Work out the finished part from the listing and answer in its coordinate system (mm). A direction names the side the tool comes from. Coordinates: 2 decimals unless noted, no trailing zeros. Order: outer loops, then holes, each group sorted by start corner. A loop starts at its lowest first (then second) coordinate and runs counter-clockwise, first axis right, second up. Notation, with made-up numbers: M -28,-36 L 15,-36 A20 ccw 15,-15 Z; hole C 16,4.25 d5. An arc over 180 degrees is marked long. Use a Markdown table: item, result.
from build123d import *

# Parameters (mm, degrees)
F0_R     = 4
F0_R_2   = 2.25
F1_DEPTH = 4
F3_DEPTH = 2
F5_R     = 2
F6_R     = 3


with BuildPart() as f1:
    # F0 (on Top) → F1 (new body)
    with BuildSketch(Plane.XY):
        with Locations((-25, 75)):
            Circle(F0_R)
        with Locations((-25, 75)):
            Circle(F0_R_2, mode=Mode.SUBTRACT)
    extrude(amount=F1_DEPTH)


with BuildPart() as f1b:
    # F0 (on Top) → F1, piece 2 (new body)
    with BuildSketch(Plane.XY):
        with Locations((25, 75)):
            Circle(F0_R)
        with Locations((25, 75)):
            Circle(F0_R_2, mode=Mode.SUBTRACT)
    extrude(amount=F1_DEPTH)


with BuildPart() as f1c:
    # F0 (on Top) → F1, piece 3 (new body)
    with BuildSketch(Plane.XY):
        with Locations((-25, -75)):
            Circle(F0_R)
        with Locations((-25, -75)):
            Circle(F0_R_2, mode=Mode.SUBTRACT)
    extrude(amount=F1_DEPTH)


with BuildPart() as f1d:
    # F0 (on Top) → F1, piece 4 (new body)
    with BuildSketch(Plane.XY):
        with Locations((25, -75)):
            Circle(F0_R)
        with Locations((25, -75)):
            Circle(F0_R_2, mode=Mode.SUBTRACT)
    extrude(amount=F1_DEPTH)


with BuildPart() as f3:
    # F2 (on Top) → F3 (new body)
    with BuildSketch(Plane.XY):
        Polygon((-22.6102852702, 72.5742723009), (-25.4563351644, 71.6255890028), (-1.5811388301, 0), (0, 4.7434164903), align=None)
        Polygon((0, 4.7434164903), (-1.5811388301, 0), (0, -4.7434164903), (1.5811388301, 0), align=None)
        Polygon((0, -4.7434164903), (-1.5811388301, 0), (-25.4563351644, -71.6255890028), (-22.6102852702, -72.5742723009), align=None)
        Polygon((1.5811388301, 0), (0, -4.7434164903), (22.6102852702, -72.5742723009), (25.4563351644, -71.6255890028), align=None)
        Polygon((22.6102852702, 72.5742723009), (0, 4.7434164903), (1.5811388301, 0), (25.4563351644, 71.6255890028), align=None)
    extrude(amount=F3_DEPTH)

    # F4: union F1d, F1c, F1b, F1
    add(f1d.part)
    add(f1c.part)
    add(f1b.part)
    add(f1.part)

    # F5
    f5_edges = [f3.edges().sort_by_distance(p)[0] for p in [
        (0, 4.743416, 1),
        (-1.581139, 0, 1),
        (0, -4.743416, 1),
        (1.581139, 0, 1),
    ]]
    fillet(f5_edges, radius=F5_R)

    # F6
    f6_edges = [f3.edges().sort_by_distance(p)[0] for p in [
        (-25.250421, 71.007847, 1),
        (-22.404371, 71.95653, 1),
        (25.250421, 71.007847, 1),
        (-22.404371, -71.95653, 1),
        (25.250421, -71.007847, 1),
        (22.404371, -71.95653, 1),
        (-25.250421, -71.007847, 1),
        (22.404371, 71.95653, 1),
    ]]
    fillet(f6_edges, radius=F6_R)


solid = f3.part
1. For faces 4 (the face through (-13.42, 35.52, 0.99)), 5 (the face through (27, -77, 4)), 6 (the face through (13.42, -35.52, 0.99)), determine the directions among +Z, -Z, +X, -X, +Y, -Y from which every point of the face is accessible in a straight line to the end or side of a thin tool.
Answers below:
| item | result |
|---|---|
| face 4 | +Z, -Z, -X |
| face 5 | +Z, +X, -X, +Y, -Y |
| face 6 | +Z, -Z, +X |
2. Section A-A on z = 1.3 is taken. Determine the outline of the cut face in (x, y).
Answers below:
| item | result |
|---|---|
| outline | M -26.47,-71.28 A4 ccw long -21.59,-72.91 A3 cw -21.88,-70.39 L -1.9,-10.44 A2 cw 1.9,-10.44 L 21.88,-70.39 A3 cw 21.59,-72.91 A4 ccw long 26.47,-71.28 A3 cw 24.73,-69.44 L 1.79,-0.63 A2 cw 1.79,0.63 L 24.73,69.44 A3 cw 26.47,71.28 A4 ccw long 21.59,72.91 A3 cw 21.88,70.39 L 1.9,10.44 A2 cw -1.9,10.44 L -21.88,70.39 A3 cw -21.59,72.91 A4 ccw long -26.47,71.28 A3 cw -24.73,69.44 L -1.79,0.63 A2 cw -1.79,-0.63 L -24.73,-69.44 A3 cw Z; hole C -25,-75 d4.5; hole C -25,75 d4.5; hole C 25,-75 d4.5; hole C 25,75 d4.5 |
3. For a pull along X with two mould halves and no side action, classify faces 1 (the face through (-23, 73, 4)), 2 (the face through (-11.75, 39.99, 0.99)), 3 (the face through (-13.099, -34.554, 0.986)) as +X half, -X half, draft (parallel to the pull), parting line (faces both ways), or undercut.
Answers below:
| item | result |
|---|---|
| face 1 | draft |
| face 2 | undercut |
| face 3 | -X half |
4. Flat-ended cylindrical pins translate along their axes: P1, Ø1.5, axis at x = 13, y = 32.5, coming from the +Z side; P2, Ø5, axis at x = -25, y = 75, coming from the -Z side. Find the tip coordinate at first contact, or state that the pin passes through.
Answers below:
| item | result |
|---|---|
| P1 | z = 2 |
| P2 | z = 0 |
5. Section B-B on y = 75 is taken. Determine the outline of the cut face in (x, z).
Answers below:
| item | result |
|---|---|
| outline | M -29,0 L -27.25,0 L -27.25,4 L -29,4 Z; M -22.75,0 L -21,0 L -21,4 L -22.75,4 Z; M 21,0 L 22.75,0 L 22.75,4 L 21,4 Z; M 27.25,0 L 29,0 L 29,4 L 27.25,4 Z |
6. Section D-D on y = -49.5 is taken. Determine the outline of the cut face in (x, z), then the cut area to 3 significant figures.
Answers below:
| item | result |
|---|---|
| outline | M -18.08,0 L -14.92,0 L -14.92,2 L -18.08,2 Z; M 14.92,0 L 18.08,0 L 18.08,2 L 14.92,2 Z |
| area | 12.6 mm² |
7. Find the intervals of material crossed by probe 1 along Y at (x, z) = (-25, 2.5); probe 2 along Y at (x, z) = (-25, 1.9); probe 3 along X at (y, z) = (-37.5, 0.55), in increasing order.
Answers below:
| item | result |
|---|---|
| probe 1 | -79 to -77.25, -72.75 to -71, 71 to 72.75, 77.25 to 79 |
| probe 2 | -79 to -77.25, -72.75 to -70.03, 70.03 to 72.75, 77.25 to 79 |
| probe 3 | -14.08 to -10.92, 10.92 to 14.08 |
8. Section C-C on x = 9.5 is taken. Determine the outline of the cut face in (y, z).
Answers below:
| item | result |
|---|---|
| outline | M -33.24,0 L -23.76,0 L -23.76,2 L -33.24,2 Z; M 23.76,0 L 33.24,0 L 33.24,2 L 23.76,2 Z |
